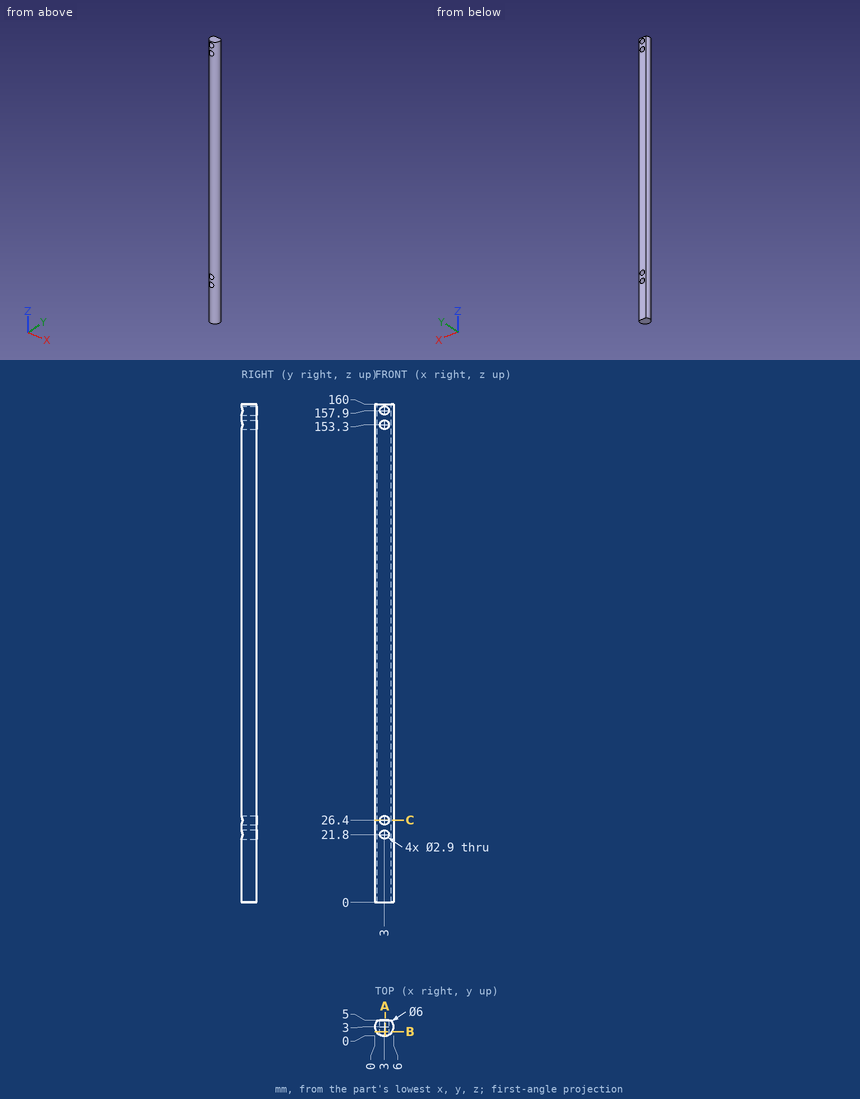
Design review of the part shown in the three views and the two pictorial views. Dimensions are in mm from the part's minimum x, y and z. Round coordinates to 2 decimals unless told otherwise and drop trailing zeros. Loops run counter-clockwise (first coordinate to the right, second up) from the corner with the lowest first, then second, coordinate; pieces in that order, holes last. Notation, with made-up numbers: (46.25, -2.75) - (67.25, -2.75) arc R23 cw to (67.25, 5.25) - close; hole circle Ø8 at (40.5, 44). An arc over 180 degrees is marked (long way). Answer as CSV lines item,"result".
(1) Insertion check: P1, Ø3, axis at x = 0.5, z = 76, coming from the -Y side; P2, Ø2, axis at x = 4.5, z = 51, coming from the -Y side; P3, Ø2.5, axis at x = 3, z = 21.8, coming from the +Y side. Each pin has a flat end and moves straight along its axis. Give the tip position at first contact, or say it passes through.
Checked values:
P1,"stops at y = 0.17"
P2,"stops at y = 0.04"
P3,"passes through"
(2) Consider section A-A on x = 3.25. Give the boundary of the cut face in (y, z).
Checked values:
outline,"(0.01, 0) - (5, 0) - (5, 20.37) - (0.01, 20.37) - close; (0.01, 23.23) - (5, 23.23) - (5, 24.97) - (0.01, 24.97) - close; (0.01, 27.83) - (5, 27.83) - (5, 151.87) - (0.01, 151.87) - close; (0.01, 154.73) - (5, 154.73) - (5, 156.47) - (0.01, 156.47) - close; (0.01, 159.33) - (5, 159.33) - (5, 160) - (0.01, 160) - close"
(3) Consider section C-C on z = 26.4. Give the boundary of the cut face in (x, y), then the cut area to 3 significant figures.
Checked values:
outline,"(0.76, 5) arc R3 ccw to (1.55, 0.37) - (1.55, 5) - close; (4.45, 0.37) arc R3 ccw to (5.24, 5) - (4.45, 5) - close"
area,"11.0 mm2"
(4) Consider section B-B on y = 1.4. Give the boundary of the cut face in (x, z), then the cut area to 3 significant figures.
Checked values:
outline,"(0.46, 0) - (5.54, 0) - (5.54, 160) - (0.46, 160) - close; hole circle Ø2.9 at (3, 21.8); hole circle Ø2.9 at (3, 26.4); hole circle Ø2.9 at (3, 153.3); hole circle Ø2.9 at (3, 157.9)"
area,"786 mm2"
(5) Wall thickness on line 1 (Z direction, x = 3.25, y = 3.8); line 2 (Z direction, x = 3.75, y = 2.35); line 3 (X direction, y = 3.2, z = 108): over which ranges is each line inside the solid? List them lowest first.
Checked values:
line 1,"z = 0 to 20.37, 23.23 to 24.97, 27.83 to 151.87, 154.73 to 156.47, 159.33 to 160"
line 2,"z = 0 to 20.56, 23.04 to 25.16, 27.64 to 152.06, 154.54 to 156.66, 159.14 to 160"
line 3,"x = 0.01 to 5.99"
